```python
from build123d import *

# Parameters (mm, degrees)
F0_W     = 12
F0_H     = 10
F1_DEPTH = 9
F2_R     = 0.95
F3_DEPTH = 10
F4_W     = 12
F4_H     = 10
F5_DEPTH = 2
F6_R     = 4
F7_DEPTH = 16


with BuildPart() as f1:
    # F0 (on Top) → F1 (new body)
    with BuildSketch(Plane.XY):
        Rectangle(F0_W, F0_H)
        with BuildLine():
            ThreePointArc((-1.939072, -1.95), (-2.75, 0), (-1.939072, 1.95))
            Line((-1.939072, 1.95), (1.939072, 1.95))
            ThreePointArc((1.939072, 1.95), (2.75, 0), (1.939072, -1.95))
            Line((1.939072, -1.95), (-1.939072, -1.95))
        make_face(mode=Mode.SUBTRACT)
    extrude(amount=F1_DEPTH)

    # F2 (on face) → F3 (cut, through all)
    with BuildSketch(Plane.XZ.offset(5)):
        with Locations((0, 5)):
            Circle(F2_R)
    extrude(amount=-F3_DEPTH, mode=Mode.SUBTRACT)

    # F4 (on face) → F5 (join)
    with BuildSketch(Plane.XY.offset(9)):
        Rectangle(F4_W, F4_H)
    extrude(amount=F5_DEPTH)

    # F6 (on face) → F7 (join)
    with BuildSketch(Plane.XY.offset(11)):
        Circle(F6_R)
    extrude(amount=F7_DEPTH)


solid = f1.part
```
The listing builds one solid part. Answer for the finished solid, in the listing's coordinates (mm). A direction names the side the tool comes from. Coordinates: 2 decimals unless noted, no trailing zeros. Loops run counter-clockwise (first coordinate to the right, second up) from the corner with the lowest first, then second, coordinate; pieces in that order, holes last. Notation, with made-up numbers: (-24.5, 32) -> (-9.5, 32) arc R16 ccw to (-9.5, 42) -> close; hole circle Ø8 at (-27.5, 36.25). An arc over 180 degrees is marked (long way). Return JSON: item names as keys, results as strings. Group by question number.
(1) A cutting plane is placed at D-D on y = -4.25. Write down the section's boundary in (x, z).
(2) A cutting plane is placed at A-A on z = 1.5. Write down the section's boundary in (x, y), and give its area (3 significant figures).
(3) Given pin 1 Ø2 at (x, y) = (1, 0.5) entering from -Z; pin 2 Ø2 at (x, z) = (-0.5, 15.5) entering from +Y; pin 3 Ø3 at (x, z) = (-4, 22.5) entering from -Y; pin 4 Ø1.5 at (x, z) = (0, 5) entering from +Y, each flat-ended and moving along its own axis, determine where each tip first touches the part or whether it passes through.
(4) Determine the mould class of faces 4 (the flat face through (-0.1, 2.3, 0)), 5 (the flat face through (6, 0, 5)), 6 (the cylindrical face through (2.75, 0.03, 4.44)), 7 (the flat face through (-6, 0, 5)) for opening direction X: released by +X, released by -X, zero draft, split by the parting line, or undercut.
(5) Find the intervals of material crossed by probe 1 along Z at (x, y) = (0, -2.7); probe 2 along Z at (x, y) = (0, 4.2); probe 3 along Y at (x, z) = (1.25, 4.75), in increasing order. Write a range as from..to.
(6) A cutting plane is placed at B-B on x = 0. Write down the section's boundary in (y, z).
(7) Which of the six approach directions +Z, -Z, +X, -X, +Y, -Y give full straight-line access (tool end or side, diameter ignored) to faces 1 (the flat face through (0, 5, 7)), 2 (the flat face through (-4.1, -1, 11)), 3 (the cylindrical face through (-2.75, -0.03, 4.44))?
(8) A cutting plane is placed at C-C on z = 5. Write down the section's boundary in (x, y).
The answers:
{
 "1": {"outline": "(-6, 0) -> (6, 0) -> (6, 11) -> (-6, 11) -> close; hole circle Ø1.9 at (0, 5)"},
 "2": {"outline": "(-6, -5) -> (6, -5) -> (6, 5) -> (-6, 5) -> close; hole (-1.94, -1.95) -> (1.94, -1.95) arc R2.75 ccw to (1.94, 1.95) -> (-1.94, 1.95) arc R2.75 ccw to start", "area": "101 mm^2"},
 "3": {"pin 1": "stops at z = 9", "pin 2": "stops at y = 4", "pin 3": "stops at y = -3.12", "pin 4": "passes through"},
 "4": {"face 4": "zero draft", "face 5": "released by +X", "face 6": "undercut", "face 7": "released by -X"},
 "5": {"probe 1": "z = 0..4.05, 5.95..27", "probe 2": "z = 0..4.05, 5.95..11", "probe 3": "y = -5..-1.95, 1.95..5"},
 "6": {"outline": "(-5, 0) -> (-1.95, 0) -> (-1.95, 4.05) -> (-5, 4.05) -> close; (-5, 5.95) -> (-1.95, 5.95) -> (-1.95, 9) -> (1.95, 9) -> (1.95, 5.95) -> (5, 5.95) -> (5, 11) -> (4, 11) -> (4, 27) -> (-4, 27) -> (-4, 11) -> (-5, 11) -> close; (1.95, 0) -> (5, 0) -> (5, 4.05) -> (1.95, 4.05) -> close"},
 "7": {"face 1": "+Z, -Z, +X, -X, +Y", "face 2": "+Z", "face 3": "-Z"},
 "8": {"outline": "(-6, -5) -> (-0.95, -5) -> (-0.95, -1.95) -> (-1.94, -1.95) arc R2.75 cw to (-1.94, 1.95) -> (-0.95, 1.95) -> (-0.95, 5) -> (-6, 5) -> close; (0.95, -5) -> (6, -5) -> (6, 5) -> (0.95, 5) -> (0.95, 1.95) -> (1.94, 1.95) arc R2.75 cw to (1.94, -1.95) -> (0.95, -1.95) -> close"}
}
